Design review of the part built by this model. Coordinates are the model's own, in mm. Face numbers are marked on the shaded views. Give positions to 0.01 mm unless a question says otherwise; leave off trailing zeros. Write each loop counter-clockwise with the first axis right and the second up, starting at its lowest first coordinate (ties: lowest second). Pieces come first, ordered by that corner, then holes.
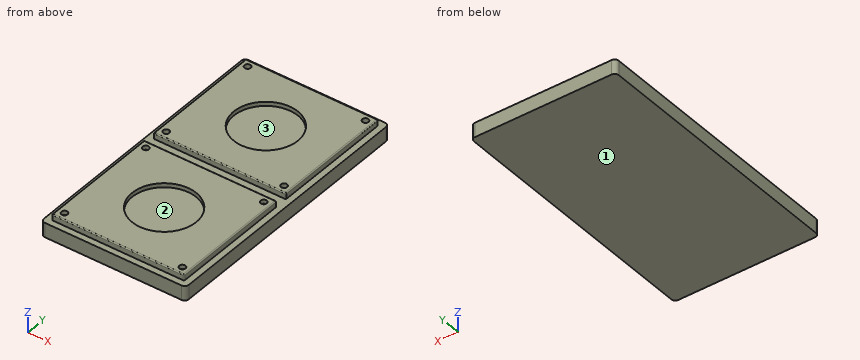
```python
from build123d import *

# Parameters (mm, degrees)
F0_W      = 70
F0_H      = 130
F1_DEPTH  = 7
F3_W      = 64
F3_H      = 59
F4_W      = 64
F4_H      = 59
F5_DEPTH  = 2.9
F7_DEPTH  = 3
F9_DEPTH  = 2
F10_R     = 0.5
F11_R     = 15.5
F12_DEPTH = 2
F13_R     = 15.5
F14_DEPTH = 2
F15_R     = 2


with BuildPart() as f1:
    # F0 (on Top) → F1 (new body)
    with BuildSketch(Plane.XY):
        with Locations((-30.63919, 34.821038)):
            Rectangle(F0_W, F0_H)
    extrude(amount=F1_DEPTH)

    # F3 (on face) + F4 (on face) → F5 (join)
    with BuildSketch(Plane.XY.offset(7)):
        with Locations((-30.63919, 67.321038)):
            Rectangle(F3_W, F3_H)
    with BuildSketch(Plane.XY.offset(7)):
        with Locations((-30.63919, 2.321038)):
            Rectangle(F4_W, F4_H)
    extrude(amount=F5_DEPTH)

    # F6 (on face) → F7 (cut)
    with BuildSketch(Plane.XY.offset(9.9)):
        with BuildLine():
            Line((-59.13919, 91.821038), (-59.13919, 93.321038))
            Line((-59.13919, 93.321038), (-57.63919, 93.321038))
            ThreePointArc((-57.63919, 93.321038), (-60.199851, 94.381698), (-59.13919, 91.821038))
        make_face()
        with BuildLine():
            Line((-57.63919, 93.321038), (-59.13919, 93.321038))
            Line((-59.13919, 93.321038), (-59.13919, 91.821038))
            ThreePointArc((-59.13919, 91.821038), (-58.07853, 92.260378), (-57.63919, 93.321038))
        make_face()
        with BuildLine():
            Line((-59.13919, 41.321038), (-59.13919, 42.821038))
            ThreePointArc((-59.13919, 42.821038), (-60.199851, 40.260378), (-57.63919, 41.321038))
            Line((-57.63919, 41.321038), (-59.13919, 41.321038))
        make_face()
        with BuildLine():
            ThreePointArc((-57.63919, 41.321038), (-58.07853, 42.381698), (-59.13919, 42.821038))
            Line((-59.13919, 42.821038), (-59.13919, 41.321038))
            Line((-59.13919, 41.321038), (-57.63919, 41.321038))
        make_face()
        with BuildLine():
            Line((-2.13919, 41.321038), (-3.63919, 41.321038))
            ThreePointArc((-3.63919, 41.321038), (-2.13919, 39.821038), (-0.63919, 41.321038))
            ThreePointArc((-0.63919, 41.321038), (-1.07853, 42.381698), (-2.13919, 42.821038))
            Line((-2.13919, 42.821038), (-2.13919, 41.321038))
        make_face()
        with BuildLine():
            ThreePointArc((-2.13919, 42.821038), (-3.199851, 42.381698), (-3.63919, 41.321038))
            Line((-3.63919, 41.321038), (-2.13919, 41.321038))
            Line((-2.13919, 41.321038), (-2.13919, 42.821038))
        make_face()
        with BuildLine():
            ThreePointArc((-0.63919, 93.321038), (-2.13919, 94.821038), (-3.63919, 93.321038))
            Line((-3.63919, 93.321038), (-2.13919, 93.321038))
            Line((-2.13919, 93.321038), (-2.13919, 91.821038))
            ThreePointArc((-2.13919, 91.821038), (-1.07853, 92.260378), (-0.63919, 93.321038))
        make_face()
        with BuildLine():
            Line((-2.13919, 93.321038), (-3.63919, 93.321038))
            ThreePointArc((-3.63919, 93.321038), (-3.199851, 92.260378), (-2.13919, 91.821038))
            Line((-2.13919, 91.821038), (-2.13919, 93.321038))
        make_face()
    extrude(amount=-F7_DEPTH, mode=Mode.SUBTRACT)

    # F8 (on face) → F9 (cut)
    with BuildSketch(Plane.XY.offset(9.9)):
        with BuildLine():
            Line((-59.13919, 28.321038), (-57.63919, 28.321038))
            ThreePointArc((-57.63919, 28.321038), (-60.199851, 29.381698), (-59.13919, 26.821038))
            Line((-59.13919, 26.821038), (-59.13919, 28.321038))
        make_face()
        with BuildLine():
            ThreePointArc((-59.13919, 26.821038), (-58.07853, 27.260378), (-57.63919, 28.321038))
            Line((-57.63919, 28.321038), (-59.13919, 28.321038))
            Line((-59.13919, 28.321038), (-59.13919, 26.821038))
        make_face()
        with BuildLine():
            Line((-59.13919, -23.678962), (-59.13919, -22.178962))
            ThreePointArc((-59.13919, -22.178962), (-60.199851, -24.739622), (-57.63919, -23.678962))
            Line((-57.63919, -23.678962), (-59.13919, -23.678962))
        make_face()
        with BuildLine():
            ThreePointArc((-57.63919, -23.678962), (-58.07853, -22.618302), (-59.13919, -22.178962))
            Line((-59.13919, -22.178962), (-59.13919, -23.678962))
            Line((-59.13919, -23.678962), (-57.63919, -23.678962))
        make_face()
        with BuildLine():
            ThreePointArc((-0.63919, 28.321038), (-2.13919, 29.821038), (-3.63919, 28.321038))
            Line((-3.63919, 28.321038), (-2.13919, 28.321038))
            Line((-2.13919, 28.321038), (-2.13919, 26.821038))
            ThreePointArc((-2.13919, 26.821038), (-1.07853, 27.260378), (-0.63919, 28.321038))
        make_face()
        with BuildLine():
            Line((-2.13919, 28.321038), (-3.63919, 28.321038))
            ThreePointArc((-3.63919, 28.321038), (-3.199851, 27.260378), (-2.13919, 26.821038))
            Line((-2.13919, 26.821038), (-2.13919, 28.321038))
        make_face()
        with BuildLine():
            ThreePointArc((-0.63919, -23.678962), (-1.07853, -22.618302), (-2.13919, -22.178962))
            Line((-2.13919, -22.178962), (-2.13919, -23.678962))
            Line((-2.13919, -23.678962), (-3.63919, -23.678962))
            ThreePointArc((-3.63919, -23.678962), (-2.13919, -25.178962), (-0.63919, -23.678962))
        make_face()
        with BuildLine():
            Line((-2.13919, -23.678962), (-2.13919, -22.178962))
            ThreePointArc((-2.13919, -22.178962), (-3.199851, -22.618302), (-3.63919, -23.678962))
            Line((-3.63919, -23.678962), (-2.13919, -23.678962))
        make_face()
    extrude(amount=-F9_DEPTH, mode=Mode.SUBTRACT)

    # F10
    f10_edges = [f1.edges().sort_by_distance(p)[0] for p in [
        (-30.63919, 37.821038, 9.9),
        (1.36081, 67.321038, 9.9),
        (1.36081, 2.321038, 9.9),
        (-30.63919, 31.821038, 9.9),
        (-30.63919, 96.821038, 9.9),
        (-62.63919, 67.321038, 9.9),
        (-62.63919, 2.321038, 9.9),
        (-30.63919, -27.178962, 9.9),
        (1.36081, -27.178962, 8.45),
        (1.36081, 31.821038, 8.45),
        (1.36081, 37.821038, 8.45),
        (1.36081, 96.821038, 8.45),
        (-62.63919, -27.178962, 8.45),
        (-62.63919, 31.821038, 8.45),
        (-62.63919, 37.821038, 8.45),
        (-62.63919, 96.821038, 8.45),
    ]]
    fillet(f10_edges, radius=F10_R)

    # F11 (on face) → F12 (cut)
    with BuildSketch(Plane.XY.offset(9.9)):
        with Locations((-30.63919, 2.321038)):
            Circle(F11_R)
    extrude(amount=-F12_DEPTH, mode=Mode.SUBTRACT)

    # F13 (on face) → F14 (cut)
    with BuildSketch(Plane.XY.offset(9.9)):
        with Locations((-30.63919, 67.321038)):
            Circle(F13_R)
    extrude(amount=-F14_DEPTH, mode=Mode.SUBTRACT)

    # F15
    f15_edges = [f1.edges().sort_by_distance(p)[0] for p in [
        (-65.63919, -30.178962, 3.5),
        (4.36081, -30.178962, 3.5),
        (4.36081, 99.821038, 3.5),
        (-65.63919, 99.821038, 3.5),
    ]]
    fillet(f15_edges, radius=F15_R)


solid = f1.part
```
(1) Consider section B-B, the plane x = -13.5. Give the boundary of the cut face in (y, z).
Resolved:
outline: (-30.18, 0) - (99.82, 0) - (99.82, 7) - (96.82, 7) - (96.82, 9.4) arc R0.5 ccw to (96.32, 9.9) - (38.32, 9.9) arc R0.5 ccw to (37.82, 9.4) - (37.82, 7) - (31.82, 7) - (31.82, 9.4) arc R0.5 ccw to (31.32, 9.9) - (-26.68, 9.9) arc R0.5 ccw to (-27.18, 9.4) - (-27.18, 7) - (-30.18, 7) - close
(2) Consider section D-D, the plane x = -33.5. Give the boundary of the cut face in (y, z), then the cut area to 3 significant figures.
Resolved:
outline: (-30.18, 0) - (99.82, 0) - (99.82, 7) - (96.82, 7) - (96.82, 9.4) arc R0.5 ccw to (96.32, 9.9) - (82.55, 9.9) - (82.55, 7.9) - (52.09, 7.9) - (52.09, 9.9) - (38.32, 9.9) arc R0.5 ccw to (37.82, 9.4) - (37.82, 7) - (31.82, 7) - (31.82, 9.4) arc R0.5 ccw to (31.32, 9.9) - (17.55, 9.9) - (17.55, 7.9) - (-12.91, 7.9) - (-12.91, 9.9) - (-26.68, 9.9) arc R0.5 ccw to (-27.18, 9.4) - (-27.18, 7) - (-30.18, 7) - close
area: 1,130 mm2
(3) Consider section A-A, the plane y = 19.5. Give the boundary of the cut face in (x, z).
Resolved:
outline: (-65.64, 0) - (4.36, 0) - (4.36, 7) - (1.36, 7) - (1.36, 9.4) arc R0.5 ccw to (0.86, 9.9) - (-62.14, 9.9) arc R0.5 ccw to (-62.64, 9.4) - (-62.64, 7) - (-65.64, 7) - close
(4) To check wall thickness, follow L1, parallel to Y at x = -30, z = 7.5; L2, parallel to Y at x = -38, z = 9; L3, parallel to Z at x = -35, y = 68. State the ranges of each line that lie inside material, in increasing order.
Resolved:
L1: y = -27.18 to 31.82, 37.82 to 96.82
L2: y = -27.18 to -11.32, 15.96 to 31.82, 37.82 to 53.68, 80.96 to 96.82
L3: z = 0 to 7.9
(5) Clearance check with flat-ended pins moving along their axes: P1, Ø1.2, axis at x = -28.5, z = 8.5, coming from the -Y side; P2, Ø2.5, axis at x = -29.5, z = 7.5, coming from the +Y side; P3, Ø1.5, axis at x = -59, y = 93, coming from the +Z side; P4, Ø2.5, axis at y = 62, z = 8.5, coming from the -X side. State where each tip first meets the part, or that it passes through.
Resolved:
P1: stops at y = -27.18
P2: stops at y = 99.82
P3: stops at z = 6.9
P4: stops at x = -62.64
(6) Mouldability with a two-part tool opening along X and no side actions: class the marked faces 1, 2 and 3 as pulls with the +X half, pulls with the -X half, needs draft (parallel to the pull), parting line crosses it, or undercut.
Resolved:
face 1: needs draft
face 2: undercut
face 3: undercut
(7) Consider section C-C, the plane y = 54. Give the boundary of the cut face in (x, z).
Resolved:
outline: (-65.64, 0) - (4.36, 0) - (4.36, 7) - (1.36, 7) - (1.36, 9.4) arc R0.5 ccw to (0.86, 9.9) - (-22.71, 9.9) - (-22.71, 7.9) - (-38.56, 7.9) - (-38.56, 9.9) - (-62.14, 9.9) arc R0.5 ccw to (-62.64, 9.4) - (-62.64, 7) - (-65.64, 7) - close
